from build123d import *

# Parameters (mm, degrees)
BOSS_EXTRUDE1_DEPTH = 6


with BuildPart() as part:
    # Sketch1 → Boss-Extrude1 (new body)
    with BuildSketch(Plane.XY):
        with BuildLine():
            Line((-38, 35), (-38, 4))
            Line((-38, 4), (-38, 3))
            Line((-38, 3), (-33.696938457, 3))
            ThreePointArc((-33.696938457, 3), (-19, 15), (-4.303061543, 3))
            Line((-4.303061543, 3), (0, 3))
            Line((0, 3), (0, 4))
            Line((0, 4), (0, 35))
            Line((0, 35), (-4, 35))
            Line((-4, 35), (-4, 41))
            Line((-4, 41), (-14, 41))
            Line((-14, 41), (-14, 35))
            Line((-14, 35), (-24, 35))
            Line((-24, 35), (-24, 41))
            Line((-24, 41), (-34, 41))
            Line((-34, 41), (-34, 35))
            Line((-34, 35), (-38, 35))
        make_face()
    extrude(amount=BOSS_EXTRUDE1_DEPTH)


solid = part.part
Model file for the job. Use its own axes, mm. A direction names the side the tool comes from. Round coordinates to 2 decimals unless told otherwise and drop trailing zeros. Loops run counter-clockwise (first coordinate to the right, second up) from the corner with the lowest first, then second, coordinate; pieces in that order, holes last.
1. Band-saw the part on B-B, the plane z = 0.55. List the corners of the cut face in (x, y), and give its area (3 significant figures).
Check values:
outline: (-38, 3) - (-33.7, 3) arc R15 cw to (-4.3, 3) - (0, 3) - (0, 35) - (-4, 35) - (-4, 41) - (-14, 41) - (-14, 35) - (-24, 35) - (-24, 41) - (-34, 41) - (-34, 35) - (-38, 35) - close
area: 1,070 mm2
2. Tool access for faces 5 (the flat face through (-36, 35, 3)), 6 (the flat face through (-2, 35, 3)), 7 (the flat face through (-19, 22, 0)), 8 (the flat face through (-24, 38, 3)), 9 (the flat face through (-36, 3, 3)): list every direction of +Z, -Z, +X, -X, +Y, -Y with a clear straight run to the whole face (end or side of a thin tool).
Check values:
face 5: +Z, -Z, -X, +Y
face 6: +Z, -Z, +X, +Y
face 7: -Z, +X, -X, +Y, -Y
face 8: +Z, -Z, +Y
face 9: +Z, -Z, +X, -X, -Y
3. Band-saw the part on D-D, the plane x = -19. List the corners of the cut face in (y, z).
Check values:
outline: (15, 0) - (35, 0) - (35, 6) - (15, 6) - close
4. Wall check: probe 1 along X at (y, z) = (36.5, 5.55); probe 2 along Y at (x, z) = (-36, 2.25); probe 3 along Y at (x, z) = (-14.5, 2.8). Give the ranges that are in metal, low to high.
Check values:
probe 1: x = -34 to -24, -14 to -4
probe 2: y = 3 to 35
probe 3: y = 14.31 to 35
5. Mould opens along X. For faces 1 (the flat face through (-14, 38, 3)), 2 (the cylindrical face through (-19, 15, 3)), 3 (the flat face through (-9, 41, 3)), 4 (the flat face through (0, 19, 3)) say: +X half, -X half, draft (parallel to the pull), parting line (faces both ways), or undercut.
Check values:
face 1: undercut
face 2: undercut
face 3: draft
face 4: +X half
6. Band-saw the part on C-C, the plane x = -34.5. List the corners of the cut face in (y, z), and give its area (3 significant figures).
Check values:
outline: (3, 0) - (35, 0) - (35, 6) - (3, 6) - close
area: 192 mm2
7. Band-saw the part on A-A, the plane y = 12.5. List the corners of the cut face in (x, z).
Check values:
outline: (-38, 0) - (-27.29, 0) - (-27.29, 6) - (-38, 6) - close; (-10.71, 0) - (0, 0) - (0, 6) - (-10.71, 6) - close
8. Drop flat-ended pins along their axis: P1, Ø6, axis at x = -13.5, y = 9.5, coming from the -Z side; P2, Ø3, axis at y = 39, z = 3.5, coming from the +X side; P3, Ø1, axis at x = -32, y = 19.5, coming from the -Z side; P4, Ø3, axis at y = 37.5, z = 2, coming from the -X side. Give the stop position or say it passes through.
Check values:
P1: passes through
P2: stops at x = -4
P3: stops at z = 0
P4: stops at x = -34
